Geometry check sheet. Reference: the model listing, model coordinates, mm. A direction names the side the tool comes from. Give positions to 0.01 mm unless a question says otherwise; leave off trailing zeros. Loops run counter-clockwise (first coordinate to the right, second up) from the corner with the lowest first, then second, coordinate; pieces in that order, holes last.
1. Material ranges on L1, parallel to Y at x = 0, z = 1.5; L2, parallel to X at y = 1.25, z = 7.75; L3, parallel to X at y = -4, z = 3.5, recorded low to high.
2. Cross-section at B-B, the plane x = 0. Record the cut outline in (y, z), plus the area to 3 significant figures.
3. Release check for a two-part mould opening along X. For faces 5 (the cylindrical face through (-0.13, 2.14, 5.45)), 6 (the flat face through (-4.5, -1, 2)), 7 (the flat face through (4.5, -1, 4)) record: +X half, -X half, draft (parallel to the pull), parting line (faces both ways), or undercut.
4. Cross-section at A-A, the plane z = 2.5. Record the cut outline in (x, y).
5. Cross-section at D-D, the plane z = 0.25. Record the cut outline in (x, y), plus the area to 3 significant figures.
6. Cross-section at C-C, the plane y = 7.25. Record the cut outline in (x, z).
7. Go/stop test with flat-tipped pins: pin 1 Ø0.6 at (x, z) = (0, -0.5) entering from -Y; pin 2 Ø3 at (x, y) = (0, 7.75) entering from -Z; pin 3 Ø2.5 at (x, y) = (-0.5, 4) entering from +Z; pin 4 Ø2 at (x, y) = (0, -7.75) entering from -Z. Record where each tip stops, or that it passes through.
8. Tool access check on faces 1 (the flat face through (0, 4.25, -1)), 2 (the flat face through (3.2, -2, 6)), 3 (the flat face through (0.9, -6.6, 0)), 4 (the flat face through (0, -5.75, 6)). Record the directions out of +Z, -Z, +X, -X, +Y, -Y that give a thin tool (end or side, any length) a straight path to the whole face; none if there is none.
from build123d import *

# Parameters (mm, degrees)
SCHIZZO1_W                   = 9
SCHIZZO1_H                   = 11.5
ESTRUSIONE_ESTRUSIONE1_DEPTH = 2
SCHIZZO2_R                   = 4.5
ESTRUSIONE_ESTRUSIONE2_DEPTH = 2
SCHIZZO3_R                   = 1.25
TAGLIO_ESTRUSIONE1_DEPTH     = 2
ESTRUSIONE_ESTRUSIONE4_DEPTH = 7.5
TAGLIO_ESTRUSIONE2_DEPTH     = 7.5
SCHIZZO7_R                   = 1
ESTRUSIONE_ESTRUSIONE5_DEPTH = 8
RACCORDO1_R                  = 1
SCHIZZO8_W                   = 9
SCHIZZO8_H                   = 9.5
ESTRUSIONE_ESTRUSIONE6_DEPTH = 2


with BuildPart() as part:
    # Schizzo1 → Estrusione-Estrusione1 (new body)
    with BuildSketch(Plane.XY):
        Rectangle(SCHIZZO1_W, SCHIZZO1_H)
    extrude(amount=ESTRUSIONE_ESTRUSIONE1_DEPTH)

    # Schizzo2 → Estrusione-Estrusione2 (add)
    with BuildSketch(Plane.XY.offset(2)):
        with Locations((0, 5.75)):
            Circle(SCHIZZO2_R)
        with Locations((0, -5.75)):
            Circle(SCHIZZO2_R)
    extrude(amount=-ESTRUSIONE_ESTRUSIONE2_DEPTH)

    # Schizzo3 → Taglio-Estrusione1 (cut)
    with BuildSketch(Plane.XY.offset(2)):
        with Locations((0, -7.75)):
            Circle(SCHIZZO3_R)
        with Locations((0, 7.75)):
            Circle(SCHIZZO3_R)
    extrude(amount=-TAGLIO_ESTRUSIONE1_DEPTH, mode=Mode.SUBTRACT)

    # Schizzo4 → Estrusione-Estrusione4 (add)
    with BuildSketch(Plane.XY.offset(2)):
        with BuildLine():
            ThreePointArc((4.5, 1.25), (0, 5.75), (-4.5, 1.25))
            Line((-4.5, 1.25), (4.5, 1.25))
        make_face()
        with BuildLine():
            Line((4.5, 1.25), (-4.5, 1.25))
            ThreePointArc((-4.5, 1.25), (0, -3.25), (4.5, 1.25))
        make_face()
        with BuildLine():
            ThreePointArc((4.5, 1.25), (0, 5.75), (-4.5, 1.25))
            Line((-4.5, 1.25), (4.5, 1.25))
        make_face()
        with BuildLine():
            Line((4.5, 1.25), (-4.5, 1.25))
            ThreePointArc((-4.5, 1.25), (0, -3.25), (4.5, 1.25))
        make_face()
        with BuildLine():
            Line((-4.5, 1.25), (-4.5, -5.75))
            Line((-4.5, -5.75), (4.5, -5.75))
            Line((4.5, -5.75), (4.5, 1.25))
            ThreePointArc((4.5, 1.25), (0, -3.25), (-4.5, 1.25))
        make_face()
    extrude(amount=ESTRUSIONE_ESTRUSIONE4_DEPTH)

    # Schizzo6 → Taglio-Estrusione2 (cut)
    with BuildSketch(Plane.XY.offset(9.5)):
        with BuildLine():
            ThreePointArc((3.2, 1.25), (0, 4.45), (-3.2, 1.25))
            Line((-3.2, 1.25), (3.2, 1.25))
        make_face()
        with BuildLine():
            Line((3.2, 1.25), (-3.2, 1.25))
            ThreePointArc((-3.2, 1.25), (0, -1.95), (3.2, 1.25))
        make_face()
        with BuildLine():
            ThreePointArc((3.2, 1.25), (0, 4.45), (-3.2, 1.25))
            Line((-3.2, 1.25), (3.2, 1.25))
        make_face()
        with BuildLine():
            Line((3.2, 1.25), (-3.2, 1.25))
            ThreePointArc((-3.2, 1.25), (0, -1.95), (3.2, 1.25))
        make_face()
        with BuildLine():
            ThreePointArc((3.2, 1.25), (0, -1.95), (-3.2, 1.25))
            Line((-3.2, 1.25), (-3.2, -4.45))
            Line((-3.2, -4.45), (3.2, -4.45))
            Line((3.2, -4.45), (3.2, 1.25))
        make_face()
    extrude(amount=-TAGLIO_ESTRUSIONE2_DEPTH, mode=Mode.SUBTRACT)

    # Schizzo7 → Estrusione-Estrusione5 (add)
    with BuildSketch(Plane.XY.offset(2)):
        with Locations((0, 1.15)):
            Circle(SCHIZZO7_R)
    extrude(amount=ESTRUSIONE_ESTRUSIONE5_DEPTH)

    # Raccordo1
    raccordo1_edges = [part.edges().sort_by_distance(p)[0] for p in [
        (-1, 1.15, 10),
    ]]
    fillet(raccordo1_edges, radius=RACCORDO1_R)

    # Schizzo8 → Estrusione-Estrusione6 (add)
    with BuildSketch(Plane(origin=(0, 0, 0), x_dir=(-1, 0, 0), z_dir=(0, 0, -1))):
        with Locations((0, -0.5)):
            Rectangle(SCHIZZO8_W, SCHIZZO8_H)
    extrude(amount=ESTRUSIONE_ESTRUSIONE6_DEPTH)


solid = part.part
Result:
1. L1: y = -10.25 to -9, -6.5 to 6.5, 9 to 10.25
1. L2: x = -4.5 to -3.2, -0.99 to 0.99, 3.2 to 4.5
1. L3: x = -4.5 to -3.2, 3.2 to 4.5
2. outline: (-10.25, 0) - (-9, 0) - (-9, 2) - (-10.25, 2) - close; (-6.5, 0) - (-5.25, 0) - (-5.25, -2) - (4.25, -2) - (4.25, 0) - (6.5, 0) - (6.5, 2) - (5.75, 2) - (5.75, 9.5) - (4.45, 9.5) - (4.45, 2) - (2.15, 2) - (2.15, 9) arc R1 ccw to (0.15, 9) - (0.15, 2) - (-4.45, 2) - (-4.45, 9.5) - (-5.75, 9.5) - (-5.75, 2) - (-6.5, 2) - close; (9, 0) - (10.25, 0) - (10.25, 2) - (9, 2) - close
2. area: 85.1 mm2
3. face 5: undercut
3. face 6: -X half
3. face 7: +X half
4. outline: (-4.5, -5.75) - (4.5, -5.75) - (4.5, 1.25) arc R4.5 ccw to (-4.5, 1.25) - close; circle Ø2 at (0, 1.15); hole (-3.2, -4.45) - (3.2, -4.45) - (3.2, 1.25) arc R3.2 ccw to (-3.2, 1.25) - close
5. outline: (-4.5, -5.75) arc R4.5 ccw to (4.5, -5.75) - (4.5, 5.75) arc R4.5 ccw to (-4.5, 5.75) - close; hole circle Ø2.5 at (0, -7.75); hole circle Ø2.5 at (0, 7.75)
5. area: 157 mm2
6. outline: (-4.24, 0) - (-1.15, 0) - (-1.15, 2) - (-4.24, 2) - close; (1.15, 0) - (4.24, 0) - (4.24, 2) - (1.15, 2) - close
7. pin 1: stops at y = -5.25
7. pin 2: stops at z = 0
7. pin 3: stops at z = 9.5
7. pin 4: passes through
8. face 1: -Z, +X, -X, +Y
8. face 2: +Z
8. face 3: -Z, +X, -X, -Y
8. face 4: +Z, +X, -X, -Y
